from build123d import *

# Parameters (mm, degrees)
SKETCH1_W           = 127
SKETCH1_H           = 50.719999906
BOSS_EXTRUDE1_DEPTH = 5
SKETCH2_W           = 5
SKETCH2_H           = 10.254787301
BOSS_EXTRUDE2_DEPTH = 5


with BuildPart() as part:
    # Sketch1 → Boss-Extrude1 (new body)
    with BuildSketch(Plane.XY):
        with Locations((0, 25.359999953)):
            Rectangle(SKETCH1_W, SKETCH1_H)
    extrude(amount=-BOSS_EXTRUDE1_DEPTH)

    # Sketch2 → Boss-Extrude2 (add)
    with BuildSketch(Plane(origin=(0, 0, -5), x_dir=(-1, 0, 0), z_dir=(0, 0, -1))):
        with Locations((-66, 12.743106261)):
            Rectangle(SKETCH2_W, SKETCH2_H)
        with Locations((-66, 37.976893645)):
            Rectangle(SKETCH2_W, SKETCH2_H)
        with Locations((66, 12.743106261)):
            Rectangle(SKETCH2_W, SKETCH2_H)
        with Locations((66, 37.976893645)):
            Rectangle(SKETCH2_W, SKETCH2_H)
    extrude(amount=-BOSS_EXTRUDE2_DEPTH)


solid = part.part
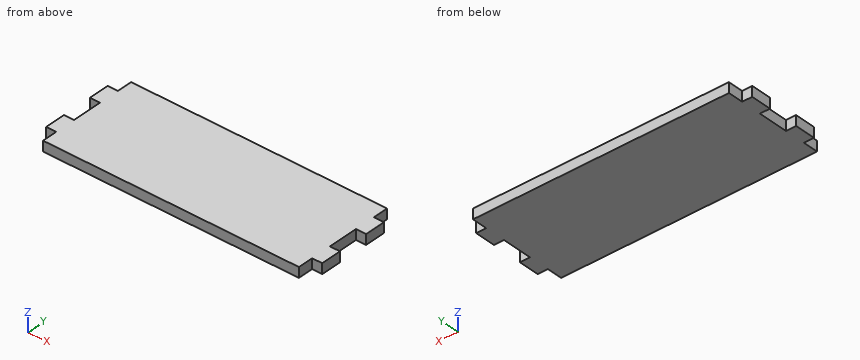
Geometry check sheet. Reference: the model listing, model coordinates, mm. Give positions to 0.01 mm unless a question says otherwise; leave off trailing zeros. Order: outer loops, then holes, each group sorted by start corner. A loop starts at its lowest first (then second) coordinate and runs counter-clockwise, first axis right, second up.
1. Sectioned sample at B-B (y = 4). Record the boundary of the cut face in (x, z).
Completed:
outline: (-63.5, -5) - (63.5, -5) - (63.5, 0) - (-63.5, 0) - close
2. Scan line: line 1 (X direction, y = 32.5, z = -0.75). Record every from-to range of solid material in increasing order.
Completed:
line 1: x = -63.5 to 63.5
3. Depth check by flat-ended pin: pin 1 (2.5 mm diameter, centred on y = 47.5, z = -3.5, fed in from +X); pin 2 (1.5 mm diameter, centred on x = -66.5, z = -1.5, fed in from +Y); pin 3 (1.5 mm diameter, centred on y = 3, z = -1.5, fed in from -X). Enter the tip coordinate at first touch or a pass-through.
Completed:
pin 1: stops at x = 63.5
pin 2: stops at y = 43.1
pin 3: stops at x = -63.5
4. Sectioned sample at A-A (z = -2.65). Record the boundary of the cut face in (x, y), then the cut area to 3 significant figures.
Completed:
outline: (-68.5, 7.62) - (-63.5, 7.62) - (-63.5, 0) - (63.5, 0) - (63.5, 7.62) - (68.5, 7.62) - (68.5, 17.87) - (63.5, 17.87) - (63.5, 32.85) - (68.5, 32.85) - (68.5, 43.1) - (63.5, 43.1) - (63.5, 50.72) - (-63.5, 50.72) - (-63.5, 43.1) - (-68.5, 43.1) - (-68.5, 32.85) - (-63.5, 32.85) - (-63.5, 17.87) - (-68.5, 17.87) - close
area: 6,650 mm2
